Geometry: final body of the model. Coordinates: model frame, mm. Give positions to 0.01 mm unless a question says otherwise; leave off trailing zeros. Put each result on its own line as item: value. Start each with the question number.
1. Section A-A on y = 67. Count the separate pieces of the cut face and the enclosed holes in it, plus the area to 3 significant figures.
2. Ray query, line 1 along Y through (x, z) = (1.65, -14); line 2 along Z through (x, y) = (3.7, 103); line 3 along Y through (x, z) = (2.2, -193). Return the intervals inside material, ascending. Write a range as from..to.
3. First-contact query: P1, Ø1.2, axis at x = 1, y = 80, coming from the +Z side; P2, Ø2, axis at x = 2, y = 53.5, coming from the +Z side; P3, Ø2, axis at x = 2.5, z = -255, coming from the -Y side. Flat tips, straight axial feed; report the tip coordinate or a pass-through.
4. Mould query, pull axis Y, two halves, no side actions, for faces 1 (the cylindrical face through (2, 10, -10)), 2 (the flat face through (4, 58, -151)). Classes: pulls with the +Y half, pulls with the -Y half, needs draft (parallel to the pull), parting line crosses it, or undercut.
from build123d import *

# Parameters (mm, degrees)
SKETCH1_W           = 307
SKETCH1_H           = 115
BOSS_EXTRUDE1_DEPTH = 4
SKETCH2_W           = 46.333333333
SKETCH2_H           = 4
BOSS_EXTRUDE2_DEPTH = 4
SKETCH3_W           = 4
SKETCH3_H           = 38
SKETCH3_H_2         = 38.5
CUT_EXTRUDE1_DEPTH  = 4
SKETCH4_W           = 4
SKETCH4_H           = 22.6
CUT_EXTRUDE2_DEPTH  = 328.856676003
SKETCH5_R           = 4
CUT_EXTRUDE3_DEPTH  = 4
LPATTERN2_COUNT     = 3
LPATTERN2_PITCH     = 84
SKETCH6_W           = 70
SKETCH6_H           = 4
BOSS_EXTRUDE3_DEPTH = 4
LPATTERN1_COUNT     = 2
LPATTERN1_PITCH     = 119
SKETCH7_W           = 18
SKETCH7_H           = 4
CUT_EXTRUDE4_DEPTH  = 4
SKETCH8_W           = 36
SKETCH8_H           = 4
BOSS_EXTRUDE5_DEPTH = 4
CUT_EXTRUDE5_DEPTH  = 4
LPATTERN3_COUNT     = 3
LPATTERN3_PITCH     = 84
LPATTERN4_COUNT     = 2
LPATTERN4_PITCH     = 110


with BuildPart() as part:
    # Sketch1 → Boss-Extrude1 (new body)
    with BuildSketch(Plane(origin=(0, 0, 0), x_dir=(0, 0, -1), z_dir=(1, 0, 0))):
        with Locations((153.5, 57.5)):
            Rectangle(SKETCH1_W, SKETCH1_H)
    extrude(amount=BOSS_EXTRUDE1_DEPTH)

    # Sketch2 → Boss-Extrude2 (add)
    with BuildSketch(Plane(origin=(4, 0, 0), x_dir=(0, 0, -1), z_dir=(1, 0, 0))):
        with Locations((23.166666667, -2)):
            Rectangle(SKETCH2_W, SKETCH2_H)
        with Locations((283.833333334, -2)):
            Rectangle(SKETCH2_W, SKETCH2_H)
    boss_extrude2 = extrude(amount=-BOSS_EXTRUDE2_DEPTH)

    # Sketch3 → Cut-Extrude1 (cut)
    with BuildSketch(Plane(origin=(4, 0, 0), x_dir=(0, 0, -1), z_dir=(1, 0, 0))):
        with Locations((2, 96)):
            Rectangle(SKETCH3_W, SKETCH3_H)
        with Locations((2, 15.25)):
            Rectangle(SKETCH3_W, SKETCH3_H_2)
    extrude(amount=-CUT_EXTRUDE1_DEPTH, mode=Mode.SUBTRACT)

    # Sketch4 → Cut-Extrude2 (cut, through all)
    with BuildSketch(Plane(origin=(4, 0, 0), x_dir=(0, 0, -1), z_dir=(1, 0, 0))):
        with Locations((255, 81.1)):
            Rectangle(SKETCH4_W, SKETCH4_H)
        with Locations((255, 35.9)):
            Rectangle(SKETCH4_W, SKETCH4_H)
    cut_extrude2 = extrude(amount=-CUT_EXTRUDE2_DEPTH, mode=Mode.SUBTRACT)

    # Sketch5 → Cut-Extrude3 (cut)
    with BuildSketch(Plane(origin=(4, 0, 0), x_dir=(0, 0, -1), z_dir=(1, 0, 0))):
        with Locations((14, 10)):
            Circle(SKETCH5_R)
    extrude(amount=-CUT_EXTRUDE3_DEPTH, mode=Mode.SUBTRACT)

    # LPattern2: Cut-Extrude2 ×3
    with Locations(*[(0, 0, i * LPATTERN2_PITCH) for i in range(1, LPATTERN2_COUNT)]):
        add(cut_extrude2, mode=Mode.SUBTRACT)

    # Sketch6 → Boss-Extrude3 (add)
    with BuildSketch(Plane.ZY):
        with Locations((-153.666666667, -2)):
            Rectangle(SKETCH6_W, SKETCH6_H)
    extrude(amount=-BOSS_EXTRUDE3_DEPTH)

    # LPattern1: Boss-Extrude2 ×2
    with Locations(*[(0, i * LPATTERN1_PITCH, 0) for i in range(1, LPATTERN1_COUNT)]):
        add(boss_extrude2)

    # Sketch7 → Cut-Extrude4 (cut)
    with BuildSketch(Plane(origin=(4, 0, 0), x_dir=(0, 0, -1), z_dir=(1, 0, 0))):
        with Locations((298, 117)):
            Rectangle(SKETCH7_W, SKETCH7_H)
    extrude(amount=-CUT_EXTRUDE4_DEPTH, mode=Mode.SUBTRACT)

    # Sketch8 → Boss-Extrude5 (add)
    with BuildSketch(Plane(origin=(4, 0, 0), x_dir=(0, 0, -1), z_dir=(1, 0, 0))):
        with Locations((271, 117)):
            Rectangle(SKETCH8_W, SKETCH8_H)
        with Locations((199, 117)):
            Rectangle(SKETCH8_W, SKETCH8_H)
        with Locations((127, 117)):
            Rectangle(SKETCH8_W, SKETCH8_H)
    extrude(amount=-BOSS_EXTRUDE5_DEPTH)

    # Sketch9 → Cut-Extrude5 (cut)
    with BuildSketch(Plane(origin=(4, 0, 0), x_dir=(0, 0, -1), z_dir=(1, 0, 0))):
        with BuildLine():
            Line((164.5, 97.5), (164.5, 17.5))
            ThreePointArc((164.5, 17.5), (162.5, 15.5), (160.5, 17.5))
            Line((160.5, 17.5), (160.5, 97.5))
            ThreePointArc((160.5, 97.5), (162.5, 99.5), (164.5, 97.5))
        make_face()
        with BuildLine():
            Line((152, 97.5), (152, 17.5))
            ThreePointArc((152, 17.5), (154, 15.5), (156, 17.5))
            Line((156, 17.5), (156, 97.5))
            ThreePointArc((156, 97.5), (154, 99.5), (152, 97.5))
        make_face()
        with BuildLine():
            Line((143.5, 97.5), (143.5, 17.5))
            ThreePointArc((143.5, 17.5), (145.5, 15.5), (147.5, 17.5))
            Line((147.5, 17.5), (147.5, 97.5))
            ThreePointArc((147.5, 97.5), (145.5, 99.5), (143.5, 97.5))
        make_face()
    cut_extrude5 = extrude(amount=-CUT_EXTRUDE5_DEPTH, mode=Mode.SUBTRACT)

    # LPattern3: Cut-Extrude5 ×3
    with Locations(*[(0, 0, -i * LPATTERN3_PITCH) for i in range(1, LPATTERN3_COUNT)]):
        add(cut_extrude5, mode=Mode.SUBTRACT)

    # LPattern4: Cut-Extrude5 ×2
    with Locations(*[(0, 0, i * LPATTERN4_PITCH) for i in range(1, LPATTERN4_COUNT)]):
        add(cut_extrude5, mode=Mode.SUBTRACT)


solid = part.part
Resolved:
1. separate pieces: 10
1. enclosed holes: 0
1. area: 1,080 mm^2
2. line 1: -4..6, 14..119
2. line 2: -307..-4
2. line 3: 0..119
3. P1: z = -4
3. P2: z = 0
3. P3: y = 0
4. face 1: undercut
4. face 2: needs draft
